Source: CAD feature listing. Evaluate the final solid. Frame: model axes, mm. Give positions to 0.01 mm unless a question says otherwise; leave off trailing zeros. Order: outer loops, then holes, each group sorted by start corner. A loop starts at its lowest first (then second) coordinate and runs counter-clockwise, first axis right, second up. Notation, with made-up numbers: M 79,-39 L 92,-39 A24 cw 92,-2 Z; hole C 60,41.25 d1. An arc over 180 degrees is marked long. Return JSON: item names as keys, results as strings.
Autodesk Inventor part; units mm, degrees
ref_plane "YZ Plane" through (0, 0, 0) normal (1, 0, 0) x (0, 1, 0)
ref_plane "XZ Plane" through (0, 0, 0) normal (0, 1, 0) x (-1, 0, 0)
ref_plane "XY Plane" through (0, 0, 0) normal (0, 0, 1) x (1, 0, 0)
sketch "Sketch1" plane through (0, 0, 0) normal (0, 0, 1) x (1, 0, 0)
  line L0 (0, 0) -> (0, 180)
  line L1 (0, 180) -> (60, 180)
  line L2 (60, 180) -> (60, 60)
  line L3 (60, 60) -> (240, 60)
  line L4 (240, 60) -> (240, 180)
  line L5 (240, 180) -> (300, 180)
  line L6 (300, 180) -> (300, 0)
  line L7 (300, 0) -> (0, 0)
  line L8 (60, 60) -> (0, 60) construction
  line L9 (60, 60) -> (60, 0) construction
  line L10 (240, 60) -> (300, 60) construction
  line L11 (240, 60) -> (240, 0) construction
  line L12 (240, 60) -> (180, 60) construction
  line L13 (180, 60) -> (180, 0) construction
  line L14 (180, 60) -> (120, 60) construction
  line L15 (120, 60) -> (120, 0) construction
  line L16 (240, 60) -> (240, 120) construction
  line L17 (240, 120) -> (300, 120) construction
  line L18 (60, 60) -> (60, 120) construction
  line L19 (60, 120) -> (0, 120) construction
  line L20 (0, 120) -> (60, 180) construction
  line L21 (0, 60) -> (60, 120) construction
  line L22 (0, 0) -> (60, 60) construction
  line L23 (60, 0) -> (120, 60) construction
  line L24 (120, 0) -> (180, 60) construction
  line L25 (180, 0) -> (240, 60) construction
  line L26 (240, 0) -> (300, 60) construction
  line L27 (240, 60) -> (300, 120) construction
  line L28 (240, 120) -> (300, 180) construction
  line L29 (5, 175) -> (55, 175) construction
  line L30 (55, 175) -> (55, 125) construction
  line L31 (55, 125) -> (5, 125) construction
  line L32 (5, 125) -> (5, 175) construction
  line L33 (5, 175) -> (55, 125) construction
  line L34 (55, 175) -> (5, 125) construction
  line L35 (5, 115) -> (55, 115) construction
  line L36 (55, 115) -> (55, 65) construction
  line L37 (55, 65) -> (5, 65) construction
  line L38 (5, 65) -> (5, 115) construction
  line L39 (5, 115) -> (55, 65) construction
  line L40 (55, 115) -> (5, 65) construction
  line L41 (5, 55) -> (55, 55) construction
  line L42 (55, 55) -> (55, 5) construction
  line L43 (55, 5) -> (5, 5) construction
  line L44 (5, 5) -> (5, 55) construction
  line L45 (5, 55) -> (55, 5) construction
  line L46 (55, 55) -> (5, 5) construction
  line L47 (65, 55) -> (115, 55) construction
  line L48 (115, 55) -> (115, 5) construction
  line L49 (115, 5) -> (65, 5) construction
  line L50 (65, 5) -> (65, 55) construction
  line L51 (65, 55) -> (115, 5) construction
  line L52 (115, 55) -> (65, 5) construction
  line L53 (125, 5) -> (175, 5) construction
  line L54 (175, 5) -> (175, 55) construction
  line L55 (175, 55) -> (125, 55) construction
  line L56 (125, 55) -> (125, 5) construction
  line L57 (125, 5) -> (175, 55) construction
  line L58 (175, 5) -> (125, 55) construction
  line L59 (185, 5) -> (235, 5) construction
  line L60 (235, 5) -> (235, 55) construction
  line L61 (235, 55) -> (185, 55) construction
  line L62 (185, 55) -> (185, 5) construction
  line L63 (185, 5) -> (235, 55) construction
  line L64 (235, 5) -> (185, 55) construction
  line L65 (245, 5) -> (295, 5) construction
  line L66 (295, 5) -> (295, 55) construction
  line L67 (295, 55) -> (245, 55) construction
  line L68 (245, 55) -> (245, 5) construction
  line L69 (245, 5) -> (295, 55) construction
  line L70 (295, 5) -> (245, 55) construction
  line L71 (295, 65) -> (245, 65) construction
  line L72 (245, 65) -> (245, 115) construction
  line L73 (245, 115) -> (295, 115) construction
  line L74 (295, 115) -> (295, 65) construction
  line L75 (295, 65) -> (245, 115) construction
  line L76 (245, 65) -> (295, 115) construction
  line L77 (245, 125) -> (295, 125) construction
  line L78 (295, 125) -> (295, 175) construction
  line L79 (295, 175) -> (245, 175) construction
  line L80 (245, 175) -> (245, 125) construction
  line L81 (245, 125) -> (295, 175) construction
  line L82 (295, 125) -> (245, 175) construction
  circle A0 centre (245, 175) radius 1.5
  circle A1 centre (295, 175) radius 1.5
  circle A2 centre (295, 125) radius 1.5
  circle A3 centre (245, 125) radius 1.5
  circle A4 centre (245, 115) radius 1.5
  circle A5 centre (295, 115) radius 1.5
  circle A6 centre (295, 65) radius 1.5
  circle A7 centre (245, 65) radius 1.5
  circle A8 centre (245, 55) radius 1.5
  circle A9 centre (295, 55) radius 1.5
  circle A10 centre (295, 5) radius 1.5
  circle A11 centre (245, 5) radius 1.5
  circle A12 centre (235, 55) radius 1.5
  circle A13 centre (185, 55) radius 1.5
  circle A14 centre (185, 5) radius 1.5
  circle A15 centre (235, 5) radius 1.5
  circle A16 centre (125, 55) radius 1.5
  circle A17 centre (175, 55) radius 1.5
  circle A18 centre (175, 5) radius 1.5
  circle A19 centre (125, 5) radius 1.5
  circle A20 centre (115, 55) radius 1.5
  circle A21 centre (65, 55) radius 1.5
  circle A22 centre (65, 5) radius 1.5
  circle A23 centre (115, 5) radius 1.5
  circle A24 centre (5, 55) radius 1.5
  circle A25 centre (55, 55) radius 1.5
  circle A26 centre (55, 5) radius 1.5
  circle A27 centre (5, 5) radius 1.5
  circle A28 centre (5, 65) radius 1.5
  circle A29 centre (55, 65) radius 1.5
  circle A30 centre (5, 115) radius 1.5
  circle A31 centre (55, 115) radius 1.5
  circle A32 centre (5, 125) radius 1.5
  circle A33 centre (55, 125) radius 1.5
  circle A34 centre (5, 175) radius 1.5
  circle A35 centre (55, 175) radius 1.5
  point P0 (30, 150)
  point P1 (30, 90)
  point P2 (30, 30)
  point P3 (90, 30)
  point P4 (150, 30)
  point P5 (210, 30)
  point P6 (270, 30)
  point P7 (270, 90)
  point P8 (270, 150)
  dimension "d0" = 180
  dimension "d1" = 60
  dimension "d2" = 120
  dimension "d3" = 180
  dimension "d4" = 60
  dimension "d5" = 60
  dimension "d6" = 60
  dimension "d7" = 60
  dimension "d8" = 60
  dimension "d9" = 50
  dimension "d10" = 50
  dimension "d11" = 50
  dimension "d12" = 50
  dimension "d13" = 50
  dimension "d14" = 50
  dimension "d15" = 50
  dimension "d16" = 50
  dimension "d17" = 50
  dimension "d18" = 50
  dimension "d19" = 50
  dimension "d20" = 50
  dimension "d21" = 50
  dimension "d22" = 50
  dimension "d23" = 50
  dimension "d24" = 50
  dimension "d25" = 50
  dimension "d26" = 50
  dimension "d27" = 3
  dimension "d28" = 3
  dimension "d29" = 3
  dimension "d30" = 3
  dimension "d31" = 3
  dimension "d32" = 3
  dimension "d33" = 3
  dimension "d34" = 3
  dimension "d35" = 3
  dimension "d36" = 3
  dimension "d37" = 3
  dimension "d38" = 3
  dimension "d39" = 3
  dimension "d40" = 3
  dimension "d41" = 3
  dimension "d42" = 3
  dimension "d43" = 3
  dimension "d44" = 3
  dimension "d45" = 3
  dimension "d46" = 3
  dimension "d47" = 3
  dimension "d48" = 3
  dimension "d49" = 3
  dimension "d50" = 3
  dimension "d51" = 3
  dimension "d52" = 3
  dimension "d53" = 3
  dimension "d54" = 3
  dimension "d55" = 3
  dimension "d56" = 3
  dimension "d57" = 3
  dimension "d58" = 3
  dimension "d59" = 3
  dimension "d60" = 3
  dimension "d61" = 3
  dimension "d62" = 3
extrude "Extrusion1" add sketch "Sketch1" along normal blind 5
fillet "Fillet1" radius 5 8 edges at (0, 180, 2.5) (60, 180, 2.5) (60, 60, 2.5) (0, 0, 2.5) (240, 60, 2.5) (300, 0, 2.5) (240, 180, 2.5) (300, 180, 2.5)
properties part number "InnerFrame"
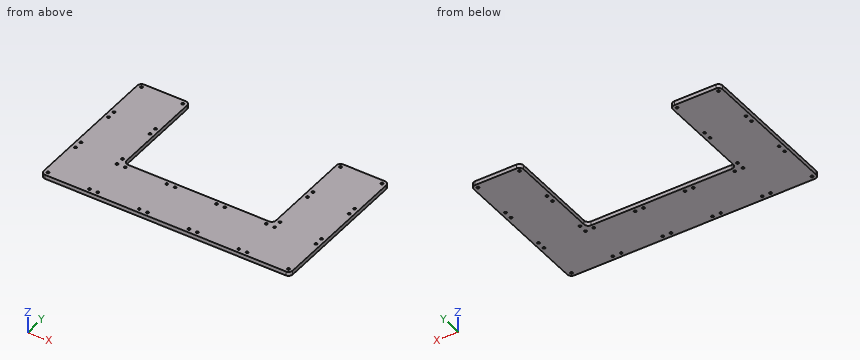
1. First-contact query: pin 1 (2.5 mm diameter, centred on x = 115, y = 55, fed in from -Z); pin 2 (1.5 mm diameter, centred on x = 150, z = 3.5, fed in from +Y). Flat tips, straight axial feed; report the tip coordinate or a pass-through.
Evaluation:
{"pin 1": "passes through", "pin 2": "stops at y = 60"}
2. Section query C-C (z = 2.8). State how many separate pieces and enclosed holes the cut face has, then the cut area to 3 significant figures.
Evaluation:
{"separate pieces": "1", "enclosed holes": "36", "area": "32,100 mm^2"}
3. Section query B-B (x = 96.5). Return loops of the section in (y, z), then the cut area to 3 significant figures.
Evaluation:
{"outline": "M 0,0 L 60,0 L 60,5 L 0,5 Z", "area": "300 mm^2"}
4. Ray query, probe 1 along X at (y, z) = (115, 0.75); probe 2 along Y at (x, z) = (185, 2.1); probe 3 along X at (y, z) = (108, 4.7). Return the intervals inside material, ascending.
Evaluation:
{"probe 1": "x = 0 to 3.5, 6.5 to 53.5, 56.5 to 60, 240 to 243.5, 246.5 to 293.5, 296.5 to 300", "probe 2": "y = 0 to 3.5, 6.5 to 53.5, 56.5 to 60", "probe 3": "x = 0 to 60, 240 to 300"}
5. Section query A-A (y = 135). Return loops of the section in (x, z), then the cut area to 3 significant figures.
Evaluation:
{"outline": "M 0,0 L 60,0 L 60,5 L 0,5 Z; M 240,0 L 300,0 L 300,5 L 240,5 Z", "area": "600 mm^2"}
